Can you work these out from the drawing? Everything is in mm from the part's minimum corner. A direction names the side the tool comes from. Coordinates: 2 decimals unless noted, no trailing zeros. Write each loop counter-clockwise with the first axis right and the second up, starting at its lowest first coordinate (ties: lowest second). Pieces come first, ordered by that corner, then holes.
(1) Thinking about a two-plate mould opening in X: for the marked faces 1, 2 and 3, which applies, released by +X, released by -X, zero draft, split by the parting line, or undercut?
(2) For pin 1 Ø4 at (y, z) = (8.5, 4.5) entering from -X, with a flat end and sliding along its axis, tell me the tip position at first contact or that it passes through.
(3) Imagine slicing it at C-C, the plane x = 40. List the corners of the cut face in (y, z) for me.
(4) Which directions (+Z, -Z, +X, -X, +Y, -Y) give clear straight access to the entire face, cutting with the end or side of a thin tool? Please do the marked faces 4 and 5.
(5) Imagine slicing it at B-B, the plane y = 5. List the corners of the cut face in (x, z) for me.
(6) Imagine slicing it at A-A, the plane z = 10. List the corners of the cut face in (x, y) for me.
(7) Please list where these lines run through material, in increasing order: probe 1 along X at (y, z) = (3, 6.75); probe 2 along Z at (x, y) = (16, 5.5).
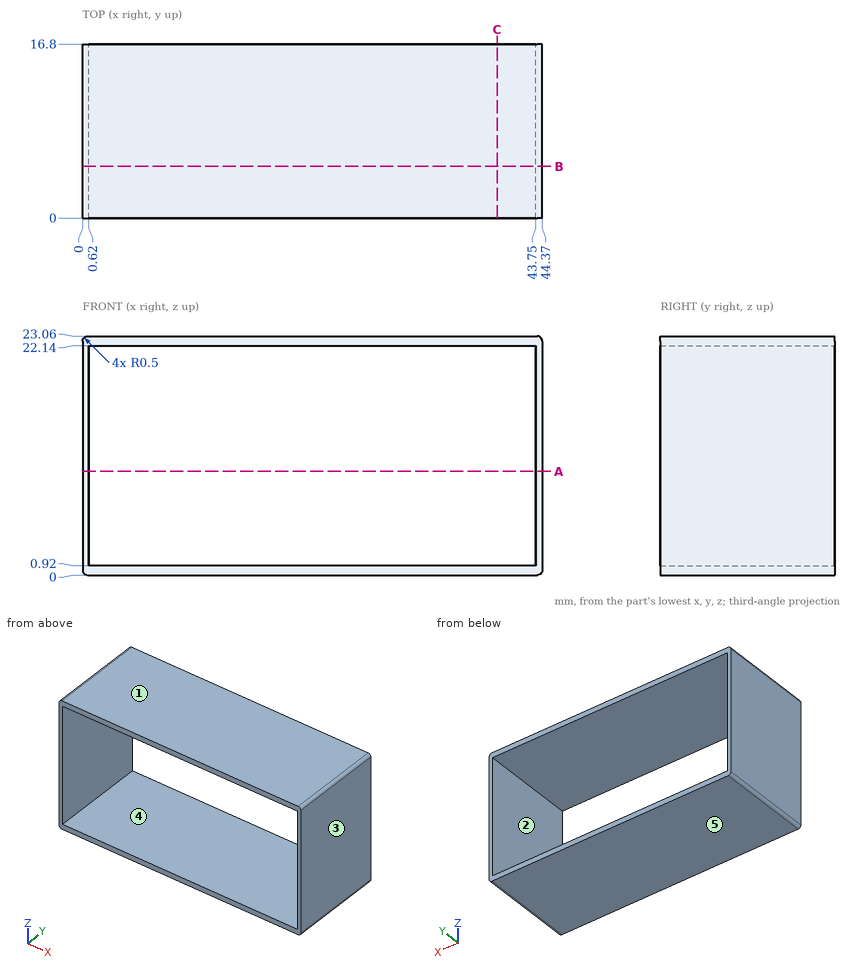
Recorded:
1. face 1: zero draft
1. face 2: undercut
1. face 3: released by +X
2. pin 1: stops at x = 0
3. outline: (0, 0) - (16.8, 0) - (16.8, 0.92) - (0, 0.92) - close; (0, 22.14) - (16.8, 22.14) - (16.8, 23.06) - (0, 23.06) - close
4. face 4: +Y, -Y
4. face 5: -Z, +X, -X, +Y, -Y
5. outline: (0, 0.5) arc R0.5 ccw to (0.5, 0) - (43.87, 0) arc R0.5 ccw to (44.37, 0.5) - (44.37, 22.56) arc R0.5 ccw to (43.87, 23.06) - (0.5, 23.06) arc R0.5 ccw to (0, 22.56) - close; hole (0.62, 0.92) - (43.75, 0.92) - (43.75, 22.14) - (0.62, 22.14) - close
6. outline: (0, 0) - (0.62, 0) - (0.62, 16.8) - (0, 16.8) - close; (43.75, 0) - (44.37, 0) - (44.37, 16.8) - (43.75, 16.8) - close
7. probe 1: x = 0 to 0.62, 43.75 to 44.37
7. probe 2: z = 0 to 0.92, 22.14 to 23.06
